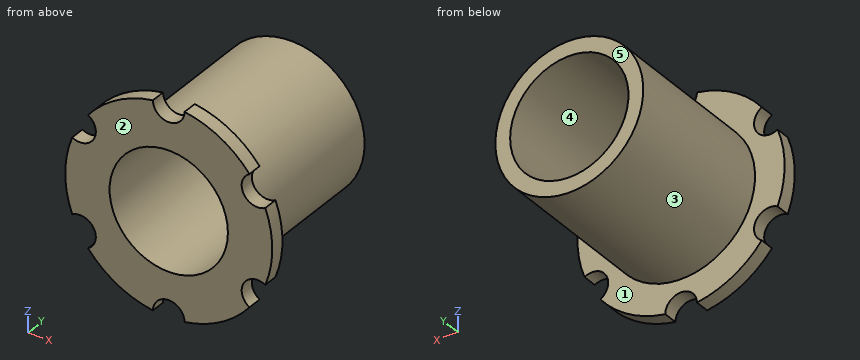
from build123d import *

# Parameters (mm, degrees)
SKETCH2_R            = 7.9375
SKETCH2_R_2          = 6.35
BOSS_EXTRUDE1_DEPTH  = 19.05
SKETCH3_R            = 11.1125
SKETCH3_R_2          = 7.9375
BOSS_EXTRUDE2_DEPTH  = 1.5875
M3_CLEARANCE_HOLE1_D = 3.4
CIRPATTERN1_COUNT    = 6


with BuildPart() as part:
    # Sketch2 → Boss-Extrude1 (new body)
    with BuildSketch(Plane(origin=(0, 0, 0), x_dir=(1, 0, 0), z_dir=(0, 1, 0))):
        Circle(SKETCH2_R)
        Circle(SKETCH2_R_2, mode=Mode.SUBTRACT)
    extrude(amount=BOSS_EXTRUDE1_DEPTH)

    # Sketch3 → Boss-Extrude2 (add)
    with BuildSketch(Plane(origin=(0, 0, 0), x_dir=(1, 0, 0), z_dir=(0, 1, 0))):
        Circle(SKETCH3_R)
        Circle(SKETCH3_R_2, mode=Mode.SUBTRACT)
    extrude(amount=BOSS_EXTRUDE2_DEPTH)

    # M3 Clearance Hole1 (through all)
    with Locations(Plane(origin=(0, 0, 0), x_dir=(-1, 0, 0), z_dir=(0, -1, 0))):
        with Locations((0, -11)):
            m3_clearance_hole1 = Hole(M3_CLEARANCE_HOLE1_D / 2)

    # CirPattern1: M3 Clearance Hole1 ×6 about axis
    cirpattern1_axis = Axis((0, 0, 0), (0, 1, 0))
    for i in range(1, CIRPATTERN1_COUNT):
        add(m3_clearance_hole1.rotate(cirpattern1_axis, i * 360 / CIRPATTERN1_COUNT), mode=Mode.SUBTRACT)


solid = part.part
The listing builds one solid part. Answer for the finished solid, in the listing's coordinates (mm). Face numbers are marked on the shaded views. A direction names the side the tool comes from. Round coordinates to 2 decimals unless told otherwise and drop trailing zeros. Order: outer loops, then holes, each group sorted by start corner. A loop starts at its lowest first (then second) coordinate and runs counter-clockwise, first axis right, second up. Notation, with made-up numbers: M 6,69 L 48,69 A21 ccw 48,104 Z; hole C 40,35 d4. An arc over 180 degrees is marked long. Answer in a Markdown table with one row per item. Add a question column.
1) Flat-ended cylindrical pins translate along their axes: pin 1 Ø2 at (x, y) = (7, 5.5) entering from -Z; pin 2 Ø5 at (y, z) = (13.5, -3.5) entering from -X; pin 3 Ø11 at (x, z) = (-4.5, -1) entering from +Y; pin 4 Ø1 at (y, z) = (14, -1) entering from +X. Find the tip coordinate at first contact, or state that the pin passes through.
2) The part is cut by section C-C on x = -8.25. Determine the outline of the cut face in (y, z).
3) Determine the mould class of the marked faces 3, 4 and 5 for opening direction X: pulls with the +X half, pulls with the -X half, needs draft (parallel to the pull), parting line crosses it, or undercut.
4) Consider line 1 along X through (y, z) = (11.75, 0); line 2 along Y through (x, z) = (-5, -8.75). Determine where each line is inside the solid, lowest interval first. Write a range as from..to.
5) The part is cut by section B-B on z = 0. Determine the outline of the cut face in (x, y).
6) The part is cut by section A-A on x = 0. Determine the outline of the cut face in (y, z).
7) Which of the six approach directions +Z, -Z, +X, -X, +Y, -Y give full straight-line access (tool end or side, diameter ignored) to the marked faces 1 and 2?
Findings below:
| question | item | result |
|---|---|---|
| 1 | pin 1 | stops at z = -5.2 |
| 1 | pin 2 | stops at x = -7.87 |
| 1 | pin 3 | stops at y = 19.05 |
| 1 | pin 4 | stops at x = 7.92 |
| 2 | outline | M 0,-7.44 L 1.59,-7.44 L 1.59,-6.62 L 0,-6.62 Z; M 0,-4.38 L 1.59,-4.38 L 1.59,4.38 L 0,4.38 Z; M 0,6.62 L 1.59,6.62 L 1.59,7.44 L 0,7.44 Z |
| 3 | face 3 | parting line crosses it |
| 3 | face 4 | undercut |
| 3 | face 5 | needs draft |
| 4 | line 1 | x = -7.94..-6.35, 6.35..7.94 |
| 4 | line 2 | y = 0..1.59 |
| 5 | outline | M -11.11,0 L -6.35,0 L -6.35,19.05 L -7.94,19.05 L -7.94,1.59 L -11.11,1.59 Z; M 6.35,0 L 11.11,0 L 11.11,1.59 L 7.94,1.59 L 7.94,19.05 L 6.35,19.05 Z |
| 6 | outline | M 0,-9.3 L 1.59,-9.3 L 1.59,-7.94 L 19.05,-7.94 L 19.05,-6.35 L 0,-6.35 Z; M 0,6.35 L 19.05,6.35 L 19.05,7.94 L 1.59,7.94 L 1.59,9.3 L 0,9.3 Z |
| 7 | face 1 | +Y |
| 7 | face 2 | +Z, -Z, +X, -X, -Y |
